from build123d import *

# Parameters (mm, degrees)
SKETCH1_W                      = 125
SKETCH1_H                      = 65
BOSS_EXTRUDE1_DEPTH            = 47
CUT_EXTRUDE1_DEPTH             = 156.312588028
SKETCH3_W                      = 30
SKETCH3_H                      = 33
CUT_EXTRUDE2_DEPTH             = 119.474680839
SKETCH4_W                      = 46
SKETCH4_H                      = 21
BOSS_EXTRUDE2_DEPTH            = 5.9
SKETCH5_W                      = 30
SKETCH5_H                      = 33
CUT_EXTRUDE3_DEPTH             = 119.474680839
SKETCH6_W                      = 46
SKETCH6_H                      = 21
BOSS_EXTRUDE3_DEPTH            = 5.9
SKETCH7_W                      = 6.4
SKETCH7_H                      = 9
CUT_EXTRUDE4_DEPTH             = 119.081539624
SKETCH8_W                      = 6.4
SKETCH8_H                      = 9
CUT_EXTRUDE5_DEPTH             = 119.081539624
SKETCH9_W                      = 8
SKETCH9_H                      = 3.5
CUT_EXTRUDE6_DEPTH             = 133.012310032
SKETCH10_W                     = 52
SKETCH10_H                     = 30.5
CUT_EXTRUDE7_DEPTH             = 8
SKETCH11_W                     = 8
SKETCH11_H                     = 3.5
CUT_EXTRUDE8_DEPTH             = 133.012310032
SKETCH12_W                     = 52
SKETCH12_H                     = 30.5
CUT_EXTRUDE9_DEPTH             = 8
SKETCH13_W                     = 33
SKETCH13_H                     = 14
CUT_EXTRUDE10_DEPTH            = 156.312588028
CUT_EXTRUDE11_DEPTH            = 156.312588028
SKETCH15_W                     = 3
SKETCH15_H                     = 3
CUT_EXTRUDE12_DEPTH            = 156.312588028
SKETCH16_W                     = 3
SKETCH16_H                     = 3
CUT_EXTRUDE13_DEPTH            = 156.312588028
F_6_8_6_8_DIAMETER_HOLE1_D     = 6.8
F_6_8_6_8_DIAMETER_HOLE1_DEPTH = 22
F_6_8_6_8_DIAMETER_HOLE1_TIP   = 2.042926105
F_6_8_6_8_DIAMETER_HOLE2_D     = 6.8
F_6_8_6_8_DIAMETER_HOLE2_DEPTH = 22
F_6_8_6_8_DIAMETER_HOLE2_TIP   = 2.042926105
F_20_0_20_DIAMETER_HOLE1_D     = 20
F_20_0_20_DIAMETER_HOLE1_DEPTH = 39
CHAMFER1_SIZE                  = 0.6
CHAMFER2_SIZE                  = 2
CHAMFER3_SIZE                  = 3.5
CHAMFER4_SIZE                  = 7
FILLET1_R                      = 3


with BuildPart() as part:
    # Sketch1 → Boss-Extrude1 (new body)
    with BuildSketch(Plane(origin=(0, 0, -23), x_dir=(-1, 0, 0), z_dir=(0, 0, -1))):
        with Locations((0, 56.5)):
            Rectangle(SKETCH1_W, SKETCH1_H)
    extrude(amount=-BOSS_EXTRUDE1_DEPTH)

    # Sketch2 → Cut-Extrude1 (cut, through all)
    with BuildSketch(Plane.ZY.offset(62.5)):
        Polygon((24, 24), (24, 63), (23, 62), (23, 24), align=None)
    extrude(amount=-CUT_EXTRUDE1_DEPTH, mode=Mode.SUBTRACT)

    # Sketch3 → Cut-Extrude2 (cut, through all)
    with BuildSketch(Plane(origin=(0, 0, -23), x_dir=(-1, 0, 0), z_dir=(0, 0, -1))):
        with Locations((47.5, 40.5)):
            Rectangle(SKETCH3_W, SKETCH3_H)
    extrude(amount=-CUT_EXTRUDE2_DEPTH, mode=Mode.SUBTRACT)

    # Sketch4 → Boss-Extrude2 (add)
    with BuildSketch(Plane.ZY.offset(32.5)):
        with Locations((0, 34.5)):
            Rectangle(SKETCH4_W, SKETCH4_H)
    extrude(amount=BOSS_EXTRUDE2_DEPTH)

    # Sketch5 → Cut-Extrude3 (cut, through all)
    with BuildSketch(Plane(origin=(0, 0, -23), x_dir=(-1, 0, 0), z_dir=(0, 0, -1))):
        with Locations((-47.5, 40.5)):
            Rectangle(SKETCH5_W, SKETCH5_H)
    extrude(amount=-CUT_EXTRUDE3_DEPTH, mode=Mode.SUBTRACT)

    # Sketch6 → Boss-Extrude3 (add)
    with BuildSketch(Plane(origin=(32.5, 0, 0), x_dir=(0, 0, -1), z_dir=(1, 0, 0))):
        with Locations((0, 34.5)):
            Rectangle(SKETCH6_W, SKETCH6_H)
    extrude(amount=BOSS_EXTRUDE3_DEPTH)

    # Sketch7 → Cut-Extrude4 (cut, through all)
    with BuildSketch(Plane.XY.offset(23)):
        with Locations((35.2, 28.5)):
            Rectangle(SKETCH7_W, SKETCH7_H)
    extrude(amount=-CUT_EXTRUDE4_DEPTH, mode=Mode.SUBTRACT)

    # Sketch8 → Cut-Extrude5 (cut, through all)
    with BuildSketch(Plane.XY.offset(23)):
        with Locations((-35.2, 28.5)):
            Rectangle(SKETCH8_W, SKETCH8_H)
    extrude(amount=-CUT_EXTRUDE5_DEPTH, mode=Mode.SUBTRACT)

    # Sketch9 → Cut-Extrude6 (cut, through all)
    with BuildSketch(Plane(origin=(32, 0, 0), x_dir=(0, 0, -1), z_dir=(1, 0, 0))):
        with Locations((-19, 25.75)):
            Rectangle(SKETCH9_W, SKETCH9_H)
    extrude(amount=-CUT_EXTRUDE6_DEPTH, mode=Mode.SUBTRACT)

    # Sketch10 → Cut-Extrude7 (cut)
    with BuildSketch(Plane.XY.offset(23)):
        with Locations((0, 42.75)):
            Rectangle(SKETCH10_W, SKETCH10_H)
    extrude(amount=-CUT_EXTRUDE7_DEPTH, mode=Mode.SUBTRACT)

    # Sketch11 → Cut-Extrude8 (cut, through all)
    with BuildSketch(Plane(origin=(32, 0, 0), x_dir=(0, 0, -1), z_dir=(1, 0, 0))):
        with Locations((19, 25.75)):
            Rectangle(SKETCH11_W, SKETCH11_H)
    extrude(amount=-CUT_EXTRUDE8_DEPTH, mode=Mode.SUBTRACT)

    # Sketch12 → Cut-Extrude9 (cut)
    with BuildSketch(Plane(origin=(0, 0, -23), x_dir=(-1, 0, 0), z_dir=(0, 0, -1))):
        with Locations((0, 42.75)):
            Rectangle(SKETCH12_W, SKETCH12_H)
    extrude(amount=-CUT_EXTRUDE9_DEPTH, mode=Mode.SUBTRACT)

    # Sketch13 → Cut-Extrude10 (cut, through all)
    with BuildSketch(Plane.ZY.offset(62.5)):
        with Locations((-6.5, 82)):
            Rectangle(SKETCH13_W, SKETCH13_H)
    extrude(amount=-CUT_EXTRUDE10_DEPTH, mode=Mode.SUBTRACT)

    # Sketch14 → Cut-Extrude11 (cut, through all)
    with BuildSketch(Plane.ZY.offset(62.5)):
        Polygon((-23, 75), (-23, 65), (-9, 65), (1, 75), align=None)
    extrude(amount=-CUT_EXTRUDE11_DEPTH, mode=Mode.SUBTRACT)

    # Sketch15 → Cut-Extrude12 (cut, through all)
    with BuildSketch(Plane.ZY.offset(62.5)):
        with Locations((11.5, 87.5)):
            Rectangle(SKETCH15_W, SKETCH15_H)
    extrude(amount=-CUT_EXTRUDE12_DEPTH, mode=Mode.SUBTRACT)

    # Sketch16 → Cut-Extrude13 (cut, through all)
    with BuildSketch(Plane.ZY.offset(62.5)):
        with Locations((22.5, 87.5)):
            Rectangle(SKETCH16_W, SKETCH16_H)
    extrude(amount=-CUT_EXTRUDE13_DEPTH, mode=Mode.SUBTRACT)

    # Ø6.8 (6.8) Diameter Hole1
    with Locations(Plane.ZY.offset(62.5)):
        with Locations((15.5, 68.6)):
            Hole(F_6_8_6_8_DIAMETER_HOLE1_D / 2, depth=F_6_8_6_8_DIAMETER_HOLE1_DEPTH)
            with Locations((0, 0, -(F_6_8_6_8_DIAMETER_HOLE1_DEPTH + F_6_8_6_8_DIAMETER_HOLE1_TIP / 2))):  # 118° drill point
                Cone(0, F_6_8_6_8_DIAMETER_HOLE1_D / 2, F_6_8_6_8_DIAMETER_HOLE1_TIP, mode=Mode.SUBTRACT)

    # Ø6.8 (6.8) Diameter Hole2
    with Locations(Plane(origin=(62.5, 0, 0), x_dir=(0, 0, -1), z_dir=(1, 0, 0))):
        with Locations((-15.5, 68.6)):
            Hole(F_6_8_6_8_DIAMETER_HOLE2_D / 2, depth=F_6_8_6_8_DIAMETER_HOLE2_DEPTH)
            with Locations((0, 0, -(F_6_8_6_8_DIAMETER_HOLE2_DEPTH + F_6_8_6_8_DIAMETER_HOLE2_TIP / 2))):  # 118° drill point
                Cone(0, F_6_8_6_8_DIAMETER_HOLE2_D / 2, F_6_8_6_8_DIAMETER_HOLE2_TIP, mode=Mode.SUBTRACT)

    # Ø20.0 (20) Diameter Hole1
    with Locations(Plane(origin=(0, 0, -15), x_dir=(-1, 0, 0), z_dir=(0, 0, -1))):
        with Locations((0, 38.65)):
            Hole(F_20_0_20_DIAMETER_HOLE1_D / 2, depth=F_20_0_20_DIAMETER_HOLE1_DEPTH)

    # Chamfer1
    chamfer1_edges = [part.edges().sort_by_distance(p)[0] for p in [
        (38.4, 33, 0),
        (-38.4, 33, 0),
        (-62.5, 68.6, 18.9),
        (62.5, 68.6, 12.1),
        (-38.4, 45, 0),
        (38.4, 45, 0),
    ]]
    chamfer(chamfer1_edges, length=CHAMFER1_SIZE)

    # Chamfer2
    chamfer2_edges = [part.edges().sort_by_distance(p)[0] for p in [
        (0, 65, -23),
    ]]
    chamfer(chamfer2_edges, length=CHAMFER2_SIZE)

    # Chamfer3
    chamfer3_edges = [part.edges().sort_by_distance(p)[0] for p in [
        (32, 24, 0),
        (-32, 24, 0),
    ]]
    chamfer(chamfer3_edges, length=CHAMFER3_SIZE)

    # Chamfer4
    chamfer4_edges = [part.edges().sort_by_distance(p)[0] for p in [
        (-62.5, 60, -23),
        (62.5, 60, -23),
    ]]
    chamfer(chamfer4_edges, length=CHAMFER4_SIZE)

    # Fillet1
    fillet1_edges = [part.edges().sort_by_distance(p)[0] for p in [
        (-26, 58, 19),
        (26, 58, 19),
        (-26, 58, -19),
        (26, 58, -19),
    ]]
    fillet(fillet1_edges, radius=FILLET1_R)


solid = part.part
The listing builds one solid part. Answer for the finished solid, in the listing's coordinates (mm). A direction names the side the tool comes from. Round coordinates to 2 decimals unless told otherwise and drop trailing zeros. Write each loop counter-clockwise with the first axis right and the second up, starting at its lowest first coordinate (ties: lowest second). Pieces come first, ordered by that corner, then holes. Notation, with made-up numbers: (72.25, -28) - (124.25, -28) arc R20 ccw to (124.25, -15) - close; hole circle Ø1 at (6.25, 64). An arc over 180 degrees is marked (long way). Use a Markdown table: item, result. Add a question column.
1. Flat-ended cylindrical pins translate along their axes: P1, Ø1.5, axis at x = -7.5, z = 12, coming from the +Y side; P2, Ø6, axis at y = 53.5, z = 4, coming from the -X side; P3, Ø1, axis at x = -44, z = -10.5, coming from the +Y side. Find the tip coordinate at first contact, or state that the pin passes through.
2. A tool of negligible diameter and unlimited length cuts with its end or side. For faces 1 (the face through (-1, 87, 21)), 2 (the face through (-1, 86, 11)), 3 (the face through (29, 27.5, 19)), from which of +Z, -Z, +X, -X, +Y, -Y can it reach the whole face along a straight path? Write none if from no direction.
3. Consider line 1 (Y direction, x = -56, z = 15.5); line 2 (Z direction, x = 13.5, y = 83.5); line 3 (Y direction, x = -41.5, z = -19). Determine where each line is inside the solid, lowest interval first.
4. The part is cut by section B-B (x = -45). Write down the section's boundary in (y, z).
5. The part is cut by section C-C (y = 38.65). Write down the section's boundary in (x, z), and give its area (3 significant figures).
6. For a pull along X with two mould halves and no side action, classify faces 4 (the face through (8, 48, 15)), 5 (the face through (0, 59, 23)), 6 (the face through (38.4, 39, 0)) as +X half, -X half, draft (parallel to the pull), parting line (faces both ways), or undercut.
7. The part is cut by section D-D (x = 4.5). Write down the section's boundary in (y, z).
8. The part is cut by section A-A (z = 7). Write down the section's boundary in (x, y), and give its area (3 significant figures).
Reported:
| question | item | result |
|---|---|---|
| 1 | P1 | y = 86 |
| 1 | P2 | x = -32.5 |
| 1 | P3 | y = 65 |
| 2 | face 1 | +Z, +X, -X, +Y |
| 2 | face 2 | -Z, +X, -X, +Y |
| 2 | face 3 | +Z, +X, -X, -Y |
| 3 | line 1 | 57 to 65.2, 72 to 89 |
| 3 | line 2 | 10 to 24 |
| 3 | line 3 | 57 to 65 |
| 4 | outline | (57, -23) - (63, -23) - (65, -21) - (65, -9) - (75, 1) - (75, 10) - (86, 10) - (86, 13) - (89, 13) - (89, 21) - (86, 21) - (86, 24) - (63, 24) - (62, 23) - (57, 23) - close; hole circle Ø6.8 at (68.6, 15.5) |
| 5 | outline | (-38.4, -23) - (-26, -23) - (-26, -15) - (-10, -15) - (-10, 15) - (-26, 15) - (-26, 23) - (-38.4, 23) - close; (10, -15) - (26, -15) - (26, -23) - (38.4, -23) - (38.4, 23) - (26, 23) - (26, 15) - (10, 15) - close |
| 5 | area | 2,100 mm^2 |
| 6 | face 4 | undercut |
| 6 | face 5 | draft |
| 6 | face 6 | +X half |
| 7 | outline | (24, -15) - (29.72, -15) - (29.72, 15) - (24, 15) - close; (47.58, -15) - (58, -15) - (58, -23) - (63, -23) - (65, -21) - (65, -9) - (75, 1) - (75, 10) - (86, 10) - (86, 13) - (89, 13) - (89, 21) - (86, 21) - (86, 24) - (63, 24) - (62, 23) - (58, 23) - (58, 15) - (47.58, 15) - close |
| 8 | outline | (-62.5, 57) - (-32.5, 57) - (-32.5, 45) - (-37.8, 45) - (-38.4, 44.4) - (-38.4, 33.6) - (-37.8, 33) - (-32, 33) - (-32, 27.5) - (-28.5, 24) - (28.5, 24) - (32, 27.5) - (32, 33) - (37.8, 33) - (38.4, 33.6) - (38.4, 44.4) - (37.8, 45) - (32.5, 45) - (32.5, 57) - (62.5, 57) - (62.5, 75) - (-62.5, 75) - close; hole circle Ø20 at (0, 38.65) |
| 8 | area | 4,200 mm^2 |
